```python
from build123d import *

# Parameters (mm, degrees)
SKETCH031_R     = 7
PAD023_DEPTH    = 12
SKETCH033_R     = 5.03
PAD024_DEPTH    = 21
PAD025_DEPTH    = 30
POCKET005_DEPTH = 5


with BuildPart() as part:
    # Sketch031 → Pad023 (new body)
    with BuildSketch(Plane.XY):
        Circle(SKETCH031_R)
    extrude(amount=PAD023_DEPTH)

    # Sketch033 → Pad024 (join)
    with BuildSketch(Plane.XY):
        Circle(SKETCH033_R)
    extrude(amount=PAD024_DEPTH)

    # Sketch034 → Pad025 (join)
    with BuildSketch(Plane.XY):
        Polygon((4.94, 0), (2.47, 4.278165), (-2.47, 4.278165), (-4.94, 0), (-2.47, -4.278165), (2.47, -4.278165), align=None)
    extrude(amount=PAD025_DEPTH)

    # Sketch032 → Pocket005 (cut)
    with BuildSketch(Plane.XY):
        Polygon((4.965, 0), (2.4825, 4.299816), (-2.4825, 4.299816), (-4.965, 0), (-2.4825, -4.299816), (2.4825, -4.299816), align=None)
    extrude(amount=POCKET005_DEPTH, mode=Mode.SUBTRACT)

    # Sketch035 → Revolution007 (revolve)
    with BuildSketch(Plane.XZ):
        Polygon((5.03, 12), (7, 12), (5.03, 14), align=None)
    revolve(axis=Axis((0, 0, 0), (0, 0, 1)))


solid = part.part
```
Geometry: final body of the model. Coordinates: model frame, mm. A direction names the side the tool comes from. Coordinates: 2 decimals unless noted, no trailing zeros. Loops run counter-clockwise (first coordinate to the right, second up) from the corner with the lowest first, then second, coordinate; pieces in that order, holes last. Notation, with made-up numbers: (50.25, 13) -> (58.25, 13) arc R27 ccw to (58.25, 35) -> close; hole circle Ø9 at (84.25, 67.5). An arc over 180 degrees is marked (long way). Use a Markdown table: item, result. Add a question column.
(1) Section query D-D, the plane z = 16. Return loops of the section in (x, y).
(2) Section query C-C, the plane z = 25. Return loops of the section in (x, y), plus the area to 3 significant figures.
(3) Pin query (flat end, axial travel): pin 1 Ø2 at (x, y) = (2, 4.5) entering from +Z; pin 2 Ø1 at (y, z) = (-2.5, 19.5) entering from -X; pin 3 Ø1 at (y, z) = (-5.5, 13) entering from -X; pin 4 Ø6 at (y, z) = (-4, 5.5) entering from +X. Return the tip coordinate at first contact, or that it passes through.
(4) Line query: line 1 along Y through (x, z) = (-3.5, 2.5); line 2 along Y through (x, z) = (-0.5, 21.25); line 3 along Z through (x, y) = (-2.25, 2.25). Output: solid intervals per line, ascending.
(5) Mould query, pull axis Y, two halves, no side actions, for faces 5 (the flat face through (-4, -2, 21)), 6 (the flat face through (3.74, 2.12, 2.46)), 7 (the flat face through (0, -4.278, 25)). Classes: pulls with the +Y half, pulls with the -Y half, needs draft (parallel to the pull), parting line crosses it, or undercut.
(6) Access query for faces 1 (the flat face through (0, 4.278, 25)), 2 (the flat face through (3.72, 2.11, 25.44)), 3 (the cylindrical face through (-0.655, 4.987, 17.451)), 4 (the flat face through (3.706, -2.18, 2.465)). Directions: +Z, -Z, +X, -X, +Y, -Y. A direction counts if a zero-diameter tool reaches every point of the face in a straight line with its end or side. Return the directions, or none.
(7) Section query B-B, the plane x = 0. Return loops of the section in (y, z).
(8) Section query A-A, the plane z = 4. Return loops of the section in (x, y) (1 decimal).
Answer:
| question | item | result |
|---|---|---|
| 1 | outline | circle Ø10.06 at (0, 0) |
| 2 | outline | (-4.94, 0) -> (-2.47, -4.28) -> (2.47, -4.28) -> (4.94, 0) -> (2.47, 4.28) -> (-2.47, 4.28) -> close |
| 2 | area | 63.4 mm^2 |
| 3 | pin 1 | stops at z = 30 |
| 3 | pin 2 | stops at x = -4.62 |
| 3 | pin 3 | stops at x = -3.75 |
| 3 | pin 4 | stops at x = 6.93 |
| 4 | line 1 | y = -6.06 to -2.54, 2.54 to 6.06 |
| 4 | line 2 | y = -4.28 to 4.28 |
| 4 | line 3 | z = 5 to 30 |
| 5 | face 5 | needs draft |
| 5 | face 6 | undercut |
| 5 | face 7 | pulls with the -Y half |
| 6 | face 1 | +Z, +X, -X, +Y |
| 6 | face 2 | +Z, +X, +Y |
| 6 | face 3 | +Z |
| 6 | face 4 | -Z |
| 7 | outline | (-7, 0) -> (-4.3, 0) -> (-4.3, 5) -> (4.3, 5) -> (4.3, 0) -> (7, 0) -> (7, 12) -> (5.03, 14) -> (5.03, 21) -> (4.28, 21) -> (4.28, 30) -> (-4.28, 30) -> (-4.28, 21) -> (-5.03, 21) -> (-5.03, 14) -> (-7, 12) -> close |
| 8 | outline | circle Ø14 at (0, 0); hole (-5, 0) -> (-2.5, -4.3) -> (2.5, -4.3) -> (5, 0) -> (2.5, 4.3) -> (-2.5, 4.3) -> close |
